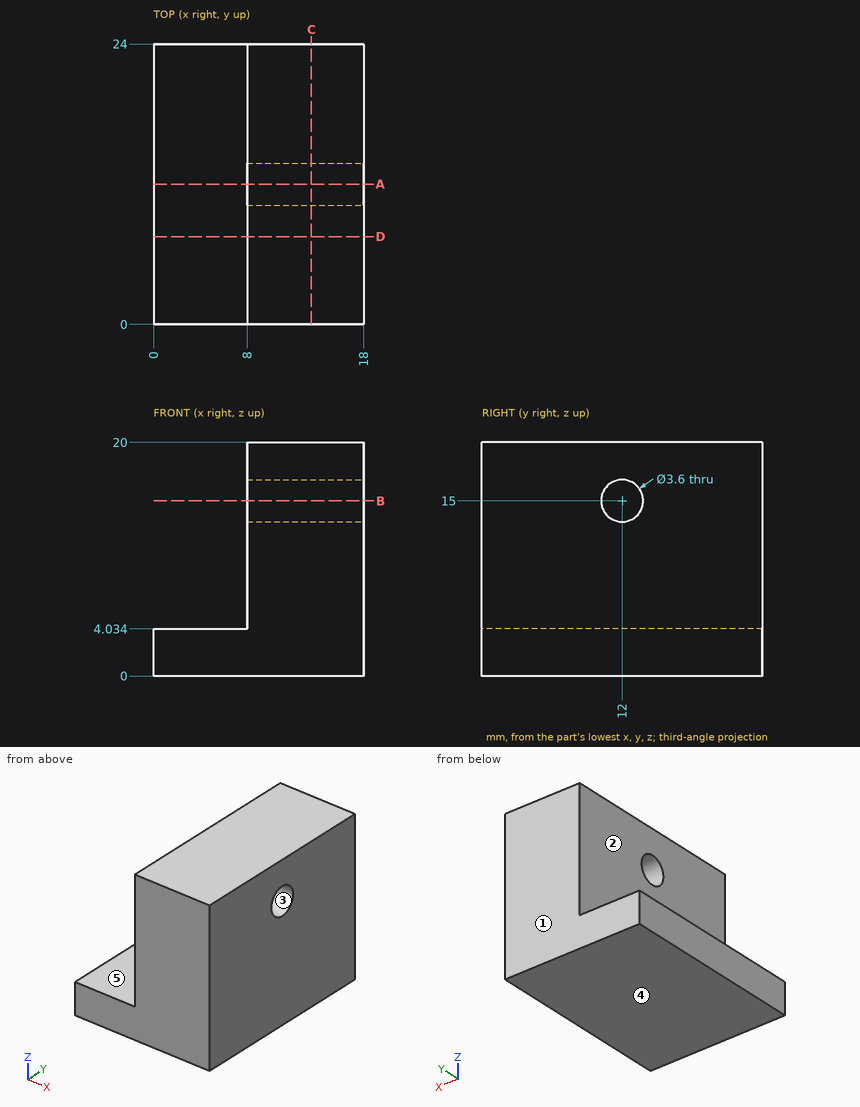
Geometry: see drawing. Coordinates: mm, zero at the bounding-box minimum. A direction names the side the tool comes from. Give positions to 0.01 mm unless a question says otherwise; leave off trailing zeros. Write each loop counter-clockwise with the first axis right and the second up, starting at its lowest first coordinate (ties: lowest second). Pieces come first, ordered by that corner, then holes. Notation, with made-up numbers: M 7,52.25 L 25,52.25 A22 cw 25,76.25 Z; hole C 17,36.5 d6. An arc over 180 degrees is marked long. Answer in a Markdown table with one row per item. Add a question column.
(1) Section B-B on z = 15. Return loops of the section in (x, y).
(2) Section A-A on y = 12. Return loops of the section in (x, z).
(3) Section D-D on y = 7.5. Return loops of the section in (x, z), and give its area (3 significant figures).
(4) Mould query, pull axis Z, two halves, no side actions, for the marked faces 3, 4 and 5. Classes: +Z half, -Z half, draft (parallel to the pull), parting line (faces both ways), or undercut.
(5) Reachability of the marked faces 1 and 2 from +Z, -Z, +X, -X, +Y, -Y: full face, straight path, thin tool, end or side. Return the list, or none.
(6) Section C-C on x = 13.5. Return loops of the section in (y, z).
(7) Ray query, line 1 (Z direction, x = 15.75, y = 12); line 2 (X direction, y = 10.5, z = 4.5); line 3 (Z direction, x = 5, y = 8). Return the intervals inside material, ascending.
(8) First-contact query: pin 1 (8 mm diameter, centred on y = 17, z = 9.5, fed in from -X); pin 2 (2.5 mm diameter, centred on x = 5.5, y = 7.5, fed in from +Z). Flat tips, straight axial feed; report the tip coordinate or a pass-through.
Result set:
| question | item | result |
|---|---|---|
| 1 | outline | M 8,0 L 18,0 L 18,10.2 L 8,10.2 Z; M 8,13.8 L 18,13.8 L 18,24 L 8,24 Z |
| 2 | outline | M 0,0 L 18,0 L 18,13.2 L 8,13.2 L 8,4.03 L 0,4.03 Z; M 8,16.8 L 18,16.8 L 18,20 L 8,20 Z |
| 3 | outline | M 0,0 L 18,0 L 18,20 L 8,20 L 8,4.03 L 0,4.03 Z |
| 3 | area | 232 mm^2 |
| 4 | face 3 | undercut |
| 4 | face 4 | -Z half |
| 4 | face 5 | +Z half |
| 5 | face 1 | +Z, -Z, +X, -X, +Y |
| 5 | face 2 | +Z, -X, +Y, -Y |
| 6 | outline | M 0,0 L 24,0 L 24,20 L 0,20 Z; hole C 12,15 d3.6 |
| 7 | line 1 | z = 0 to 13.2, 16.8 to 20 |
| 7 | line 2 | x = 8 to 18 |
| 7 | line 3 | z = 0 to 4.03 |
| 8 | pin 1 | stops at x = 8 |
| 8 | pin 2 | stops at z = 4.03 |
